The model under review builds one solid part; all positions refer to its coordinate system, in mm. Face numbers are marked on the shaded views. A direction names the side the tool comes from. Give positions to 0.01 mm unless a question says otherwise; leave off trailing zeros. Order: outer loops, then holes, each group sorted by start corner. A loop starts at its lowest first (then second) coordinate and runs counter-clockwise, first axis right, second up.
```python
from build123d import *

# Parameters (mm, degrees)
F0_R     = 4
F1_DEPTH = 10
F2_R     = 3
F3_DEPTH = 10


with BuildPart() as f1:
    # F0 (on Front) → F1 (new body)
    with BuildSketch(Plane.XZ):
        Polygon((-20, 30), (-20, 0), (20, 0), (20, 30), (9.614969, 42), (-9.72316, 42), align=None)
        with Locations((0, 27)):
            Circle(F0_R, mode=Mode.SUBTRACT)
    extrude(amount=-F1_DEPTH)

    # F2 (on face) → F3 (cut)
    with BuildSketch(Plane(origin=(0, 0, 0), x_dir=(1, 0, 0), z_dir=(0, 0, -1))):
        with Locations((-15, -5)):
            Circle(F2_R)
        with Locations((15, -5)):
            Circle(F2_R)
    extrude(amount=-F3_DEPTH, mode=Mode.SUBTRACT)


solid = f1.part
```
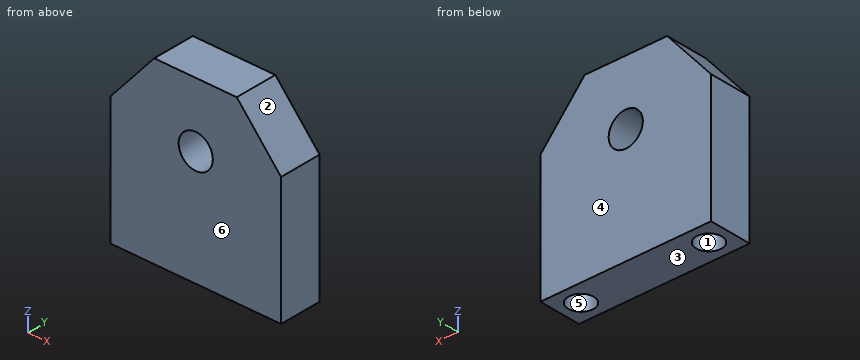
Item 1: Take a section at A-A (x = 0). Give the boundary of the cut face in (y, z), and give its area (3 significant figures).
Values found:
outline: (0, 0) - (10, 0) - (10, 23) - (0, 23) - close; (0, 31) - (10, 31) - (10, 42) - (0, 42) - close
area: 340 mm2
Item 2: Clearance check with a flat-ended pin moving along its axis: pin 1 Ø5 at (x, y) = (15, 5) entering from -Z. State where the tip first meets the part, or that it passes through.
Values found:
pin 1: stops at z = 10
Item 3: Draft analysis for pull direction Y (two halves, no side actions). For the marked faces 3, 4, 5 and 6, state which applies: released by +Y, released by -Y, zero draft, split by the parting line, or undercut.
Values found:
face 3: zero draft
face 4: released by +Y
face 5: undercut
face 6: released by -Y
Item 4: Take a section at B-B (y = 5). Give the boundary of the cut face in (x, z), and give its area (3 significant figures).
Values found:
outline: (-20, 0) - (-18, 0) - (-18, 10) - (-12, 10) - (-12, 0) - (12, 0) - (12, 10) - (18, 10) - (18, 0) - (20, 0) - (20, 30) - (9.61, 42) - (-9.72, 42) - (-20, 30) - close; hole circle Ø8 at (0, 27)
area: 1,390 mm2
Item 5: Take a section at C-C (z = 27). Give the boundary of the cut face in (x, y), and give its area (3 significant figures).
Values found:
outline: (-20, 0) - (-4, 0) - (-4, 10) - (-20, 10) - close; (4, 0) - (20, 0) - (20, 10) - (4, 10) - close
area: 320 mm2
Item 6: Take a section at D-D (z = 9). Give the boundary of the cut face in (x, y), and give its area (3 significant figures).
Values found:
outline: (-20, 0) - (20, 0) - (20, 10) - (-20, 10) - close; hole circle Ø6 at (-15, 5); hole circle Ø6 at (15, 5)
area: 343 mm2
Item 7: For line 1 (X direction, y = 5, z = 3.75); line 2 (Y direction, x = 15, z = 5); line 3 (Z direction, x = 0, y = 2.5), list the stretches that pass through material, from the lowest coordinate up.
Values found:
line 1: x = -20 to -18, -12 to 12, 18 to 20
line 2: y = 0 to 2, 8 to 10
line 3: z = 0 to 23, 31 to 42
Item 8: For the marked faces 1 and 2, list the 3-axis set-ups (+Z, -Z, +X, -X, +Y, -Y) from which the entire face can be reached by the end or side of a thin tool; tool diameter is ignored.
Values found:
face 1: -Z
face 2: +Z, +X, +Y, -Y
